Geometry check sheet. Reference: the model listing, model coordinates, mm. A direction names the side the tool comes from. Coordinates: 2 decimals unless noted, no trailing zeros. Write each loop counter-clockwise with the first axis right and the second up, starting at its lowest first coordinate (ties: lowest second). Pieces come first, ordered by that corner, then holes. Notation, with made-up numbers: (-29.5, 71.5) -> (0.5, 71.5) arc R17 ccw to (0.5, 103.5) -> close; hole circle Ø10 at (8.5, 24). An arc over 180 degrees is marked (long way). Put each result on its own line as item: value. Start each with the question number.
from build123d import *

# Parameters (mm, degrees)
SKETCH1_W        = 200
SKETCH1_H        = 210
SKETCH1_W_2      = 191
SKETCH1_H_2      = 201
SKETCH1_W_3      = 5
SKETCH1_H_3      = 2.5
SKETCH1_W_4      = 2.5
SKETCH1_H_4      = 5
MAINBODY_DEPTH   = 50
IRHOLE_START     = -4.5
IRHOLE_OUTLINE_W = 144
IRHOLE_OUTLINE_H = 25
IRHOLE_DEPTH     = 4.5


# Read off the part's stored shape, not the designer's step: IRHole
with BuildPart() as part:
    # Sketch1 → MainBody (new body)
    with BuildSketch(Plane(origin=(0, 0, 0), x_dir=(1, 0, 0), z_dir=(0, 1, 0))):
        Rectangle(SKETCH1_W, SKETCH1_H)
        Rectangle(SKETCH1_W_2, SKETCH1_H_2, mode=Mode.SUBTRACT)
        with Locations((93.5, -102.75)):
            Rectangle(SKETCH1_W_3, SKETCH1_H_3, mode=Mode.SUBTRACT)
        with Locations((0, -102.75)):
            Rectangle(SKETCH1_W_3, SKETCH1_H_3, mode=Mode.SUBTRACT)
        with Locations((-93.5, -102.75)):
            Rectangle(SKETCH1_W_3, SKETCH1_H_3, mode=Mode.SUBTRACT)
        with Locations((-83.25, 102.75)):
            Rectangle(SKETCH1_W_3, SKETCH1_H_3, mode=Mode.SUBTRACT)
        with Locations((85.75, 102.75)):
            Rectangle(SKETCH1_W_3, SKETCH1_H_3, mode=Mode.SUBTRACT)
        with Locations((97.75, -47.5)):
            Rectangle(SKETCH1_W_4, SKETCH1_H_4, mode=Mode.SUBTRACT)
        with Locations((97.75, 47.5)):
            Rectangle(SKETCH1_W_4, SKETCH1_H_4, mode=Mode.SUBTRACT)
        with Locations((-97.75, -47.5)):
            Rectangle(SKETCH1_W_4, SKETCH1_H_4, mode=Mode.SUBTRACT)
        with Locations((-97.75, 47.5)):
            Rectangle(SKETCH1_W_4, SKETCH1_H_4, mode=Mode.SUBTRACT)
    extrude(amount=MAINBODY_DEPTH)

    # IRHole outline → IRHole (cut)
    with BuildSketch(Plane(origin=(0, 0, -105), x_dir=(-1, 0, 0), z_dir=(0, 0, -1)).offset(IRHOLE_START)):
        with Locations((0, 12.5)):
            Rectangle(IRHOLE_OUTLINE_W, IRHOLE_OUTLINE_H)
    extrude(amount=IRHOLE_DEPTH, mode=Mode.SUBTRACT)


solid = part.part
Item 1: Access from +Z, -Z, +X, -X, +Y, -Y to the whole of each face (thin tool, end or side, straight path). Record for faces 1 (the flat face through (-1, 36, -100.5)), 2 (the flat face through (-1, 25, 105)), 3 (the flat face through (-72, 12, -103)).
Item 2: Mould release check, pull along Z, two halves, no side actions. Record for faces 4 (the flat face through (1, 25, -103)), 5 (the flat face through (-99, 25, 48)), 6 (the flat face through (-1, 36, -105)): released by +Z, released by -Z, zero draft, split by the parting line, or undercut.
Item 3: Section check D-D, the plane y = 32.5. Give the number of separate pieces and of enclosed holes in the cut face, and give its area (3 significant figures).
Item 4: Scan lines: line 1 along X through (y, z) = (30.5, -48); line 2 along X through (y, z) = (25, 93); line 3 along Z through (x, y) = (-40, 46). Record each from-to range of solid material in increasing order. Write a range as [from, to].
Item 5: Section check C-C, the plane z = -47.5. Enter the section's corners in (x, y).
Item 6: Section check B-B, the plane x = -18. Enter the section's corners in (y, z), and give its area (4 significant figures).
Item 7: Section check A-A, the plane z = -73. Enter the section's corners in (x, y), and give its area (3 significant figures).
From the geometry:
1. face 1: +Y, -Y
1. face 2: +Z, +X, -X, +Y, -Y
1. face 3: -Z, -Y
2. face 4: zero draft
2. face 5: undercut
2. face 6: released by -Z
3. separate pieces: 1
3. enclosed holes: 10
3. area: 3,500 mm²
4. line 1: [-100, -99], [-96.5, -95.5], [95.5, 96.5], [99, 100]
4. line 2: [-100, -95.5], [95.5, 100]
4. line 3: [-105, -100.5], [100.5, 105]
5. outline: (-100, 0) -> (-99, 0) -> (-99, 50) -> (-100, 50) -> close; (-96.5, 0) -> (-95.5, 0) -> (-95.5, 50) -> (-96.5, 50) -> close; (95.5, 0) -> (96.5, 0) -> (96.5, 50) -> (95.5, 50) -> close; (99, 0) -> (100, 0) -> (100, 50) -> (99, 50) -> close
6. outline: (0, 100.5) -> (50, 100.5) -> (50, 105) -> (0, 105) -> close; (25, -105) -> (50, -105) -> (50, -100.5) -> (25, -100.5) -> close
6. area: 337.5 mm²
7. outline: (-100, 0) -> (-95.5, 0) -> (-95.5, 50) -> (-100, 50) -> close; (95.5, 0) -> (100, 0) -> (100, 50) -> (95.5, 50) -> close
7. area: 450 mm²
